Geometry: see drawing. Coordinates: mm, zero at the bounding-box minimum. A direction names the side the tool comes from. Coordinates: 2 decimals unless noted, no trailing zeros. Loops run counter-clockwise (first coordinate to the right, second up) from the corner with the lowest first, then second, coordinate; pieces in that order, holes last. Notation, with made-up numbers: (59.5, 35) -> (68.5, 35) arc R20 cw to (68.5, 74) -> close; hole circle Ø7 at (-2.75, 42.5). An arc over 180 degrees is marked (long way). Put each result on its own line as item: value. Start each with the question number.
1) Pull-direction query (Z, two-part tool) for the marked faces 6, 7 and 8; classes: pulls with the +Z half, pulls with the -Z half, needs draft (parallel to the pull), parting line crosses it, or undercut.
2) Cut plane A-A (z = 26.5). State how many separate pieces and enclosed holes the cut face has, plus the area to 3 significant figures.
3) Cut plane B-B (x = 109). Return the cut outline in (y, z).
4) Set-up query: the marked faces 1, 2, 3, 4 and 5. Return all of +Z, -Z, +X, -X, +Y, -Y with unobstructed straight access to the full face (end or side cutting, diameter ignored); none if empty.
5) Material intervals for L1, parallel to Z at x = 71.5, y = 14; L2, parallel to X at y = 14.25, z = 27.94 (1 decimal); L3, parallel to Z at x = 25, y = 10, sorted ascending.
6) Contact query for flat-ended pins moving along their axis: P1, Ø6, axis at y = 8, z = 79.5, coming from the +X side; P2, Ø10, axis at y = 8, z = 34, coming from the -X side; P3, Ø5.5, axis at x = 183.5, y = 12, coming from the -Z side; P4, Ø8, axis at x = 133, z = 88, coming from the +Y side. Output: stop coordinate, or through.
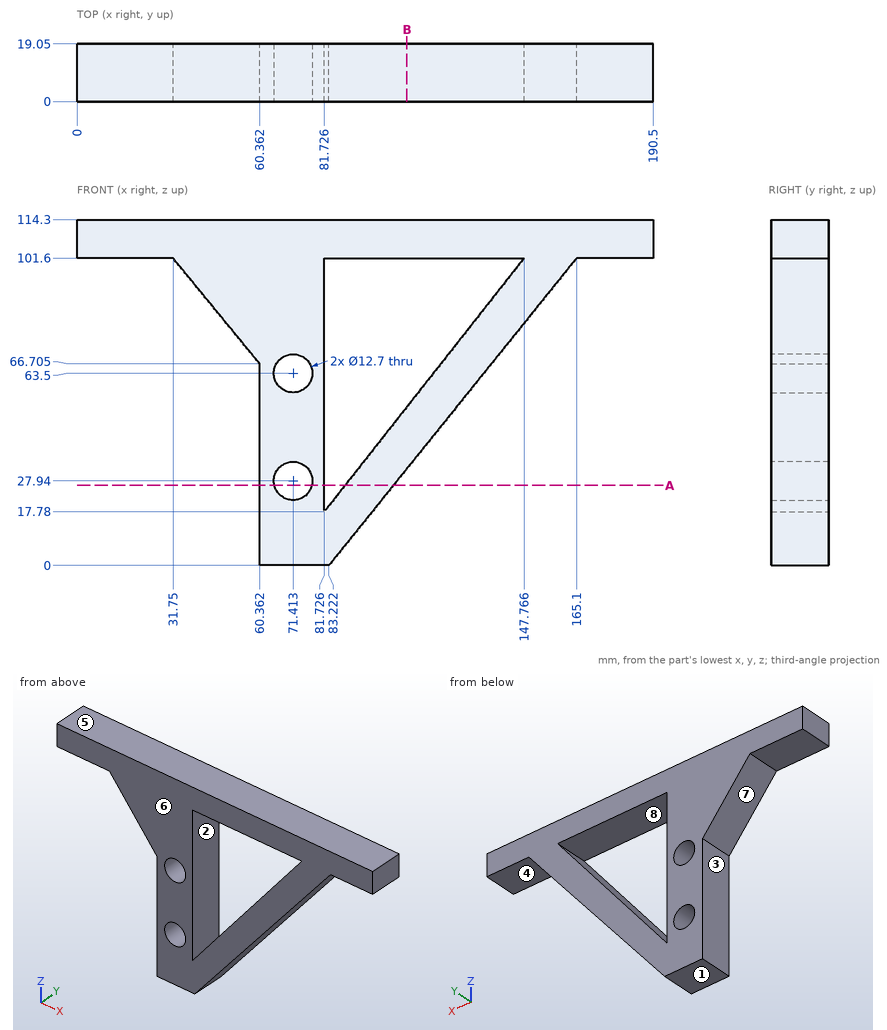
Results found:
1. face 6: needs draft
1. face 7: pulls with the -Z half
1. face 8: undercut
2. separate pieces: 3
2. enclosed holes: 0
2. area: 476 mm2
3. outline: (0, 31.99) -> (19.05, 31.99) -> (19.05, 52.4) -> (0, 52.4) -> close; (0, 101.6) -> (19.05, 101.6) -> (19.05, 114.3) -> (0, 114.3) -> close
4. face 1: -Z, +X, -X, +Y, -Y
4. face 2: +Y, -Y
4. face 3: -Z, -X, +Y, -Y
4. face 4: -Z, +X, +Y, -Y
4. face 5: +Z, +X, -X, +Y, -Y
5. L1: z = 0 to 21.59, 34.29 to 57.15, 69.85 to 114.3
5. L2: x = 60.4 to 65.1, 77.8 to 81.7, 89.7 to 105.7
5. L3: z = 101.6 to 114.3
6. P1: stops at x = 149.71
6. P2: stops at x = 60.36
6. P3: stops at z = 101.6
6. P4: stops at y = 19.05
